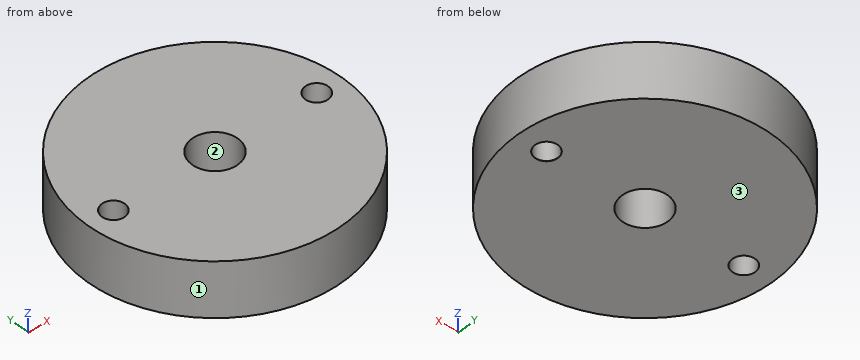
Autodesk Inventor part; units mm, degrees
ref_plane "YZ Plane" through (0, 0, 0) normal (1, 0, 0) x (0, 1, 0)
ref_plane "XZ Plane" through (0, 0, 0) normal (0, 1, 0) x (-1, 0, 0)
ref_plane "XY Plane" through (0, 0, 0) normal (0, 0, 1) x (1, 0, 0)
sketch "Sketch1" plane through (0, 0, 0) normal (0, 0, 1) x (1, 0, 0)
  circle A0 centre (0, 0) radius 7
  dimension "d0" = 14
extrude "Extrusion1" add sketch "Sketch1" along normal blind 3
sketch "Sketch2" plane through (0, 0, 3) normal (0, 0, 1) x (1, 0, 0)
  circle A0 centre (0, 0) radius 1.25
  dimension "d3" = 2.5
extrude "Extrusion2" cut sketch "Sketch2" against normal blind 3
sketch "Sketch3" plane through (0, 0, 3) normal (0, 0, 1) x (1, 0, 0)
  circle A0 centre (-5.575, 0) radius 0.625
  circle A1 centre (0, 0) radius 7
  circle A2 centre (5.575, 0) radius 0.625
  dimension "d6" = 1.25
  dimension "d7" = 1.25
  dimension "d9" = 0.8
  dimension "d10" = 0.8
  dimension "d12" = 9.9
sketch "Sketch4" plane through (0, 0, 0) normal (0, 1, 0) x (-1, 0, 0)
  line L0 (7, 3) -> (-7, 3)
  line L1 (5.5663, 3) -> (5.4, -0.2434)
  line L2 (7, 0) -> (7, 3)
  point P0 (0, 0)
  dimension "d13" = 1.6
sweep "Sweep1" cut profiles "Sketch3" path "Sketch4" path curves L1 contours A0
sketch "Sketch5" plane through (0, 0, 3) normal (0, 0, 1) x (1, 0, 0)
  circle A0 centre (5.5837, 0) radius 0.625
  circle A1 centre (-5.5663, 0) radius 0.625
  point P0 (0, 0)
  dimension "d16" = 1.25
  dimension "d17" = 9.9
sketch "Sketch6" plane through (0, 0, 0) normal (0, 1, 0) x (-1, 0, 0)
  line L0 (-5.575, 2.9594) -> (-5.4, 0)
  line L1 (-7, 0) -> (7, 0)
  line L2 (-7, 0) -> (-7, 3)
  line L3 (-5.4, 0) -> (-5.4, -0.6456)
  point P0 (0, 0)
  dimension "d18" = 1.425
  dimension "d19" = 1.6
sweep "Sweep2" cut profiles "Sketch5" path "Sketch6" path curves L0 L3 contours A0
properties part number "MUSAB6" material "Bronze"
Could you check a few things on this model? Use its own coordinates, in mm. Face numbers are marked on the shaded views. Give positions to 0.01 mm unless a question says otherwise; leave off trailing zeros. Write each loop counter-clockwise with the first axis right and the second up, starting at its lowest first coordinate (ties: lowest second). Pieces come first, ordered by that corner, then holes. Notation, with made-up numbers: (24.5, 80.25) - (78.5, 80.25) arc R8 ccw to (78.5, 95.25) - close; hole circle Ø2 at (67.5, 7). An arc over 180 degrees is marked (long way). Use CSV: the item, a comma, the result in double quotes. Start each with the question number.
Item 1: If we mould it in two halves opening along X, with no side actions, what happens to the marked faces 1, 2 and 3? For each: pulls with the +X half, pulls with the -X half, needs draft (parallel to the pull), parting line crosses it, or undercut.
Item 2: I want a section at C-C, the plane x = -2.5. Please give me the cut outline in (y, z).
Item 3: I want a section at A-A, the plane x = 0. Please give me the cut outline in (y, z).
Item 4: If I drill on line 1 along Y through (x, z) = (0, 1.8); line 2 along Y through (x, z) = (-1, 2.35); line 3 along Y through (x, z) = (-2, 1.2), over which ranges is the centre line in solid material (lowest first)?
Item 5: I want a section at B-B, the plane y = 0. Give the number of separate pieces and of enclosed holes in the cut face, then the cut area to 3 significant figures.
Item 6: I'm going to push a flat-ended pin straight in: pin 1 (1.5 mm diameter, centred on x = 4.5, z = 1, fed in from -Y). Where does the tip first touch, or does it pass through?
Item 7: I want a section at D-D, the plane y = -2.25. Please give me the cut outline in (x, z).
Findings:
1,face 1,"parting line crosses it"
1,face 2,"undercut"
1,face 3,"needs draft"
2,outline,"(-6.54, 0) - (6.54, 0) - (6.54, 3) - (-6.54, 3) - close"
3,outline,"(-7, 0) - (-1.25, 0) - (-1.25, 3) - (-7, 3) - close; (1.25, 0) - (7, 0) - (7, 3) - (1.25, 3) - close"
4,line 1,"y = -7 to -1.25, 1.25 to 7"
4,line 2,"y = -6.93 to -0.75, 0.75 to 6.93"
4,line 3,"y = -6.71 to 6.71"
5,separate pieces,"4"
5,enclosed holes,"0"
5,area,"27.0 mm2"
6,pin 1,"stops at y = -5.91"
7,outline,"(-6.63, 0) - (6.63, 0) - (6.63, 3) - (-6.63, 3) - close"
